Here's the drawing with two shaded views (mm, measured from the low corner). I have some questions. A direction names the side the tool comes from. Coordinates: 2 decimals unless noted, no trailing zeros. Write each loop counter-clockwise with the first axis right and the second up, starting at its lowest first coordinate (ties: lowest second). Pieces come first, ordered by that corner, then holes. Notation, with made-up numbers: (18.25, -17.75) -> (31.25, -17.75) arc R24 ccw to (31.25, 10.25) -> close; hole circle Ø4 at (76, 8). An arc over 180 degrees is marked (long way). Use one line per item in the form item = value.
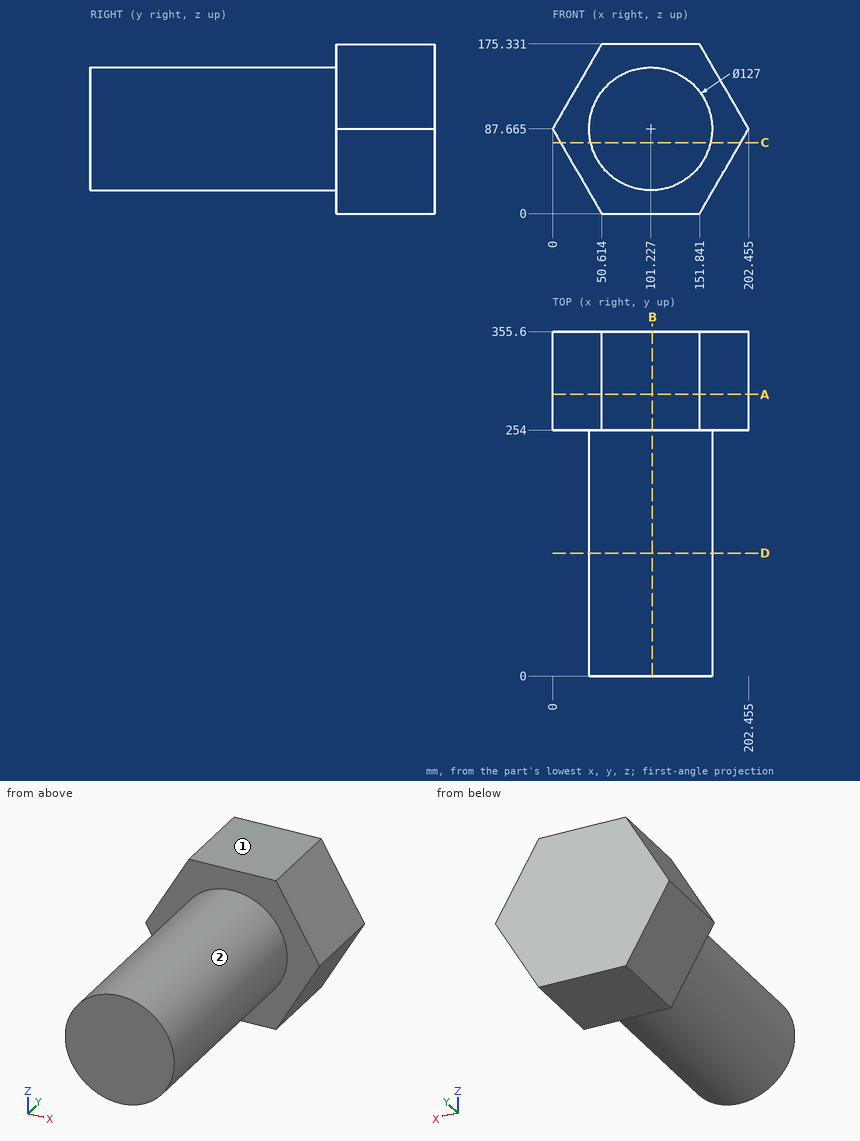
Q1. Suppose I cut it at B-B (x = 103). Write out the boundary of the cut face in (y, z).
Return value:
outline = (0, 24.19) -> (254, 24.19) -> (254, 0) -> (355.6, 0) -> (355.6, 175.33) -> (254, 175.33) -> (254, 151.14) -> (0, 151.14) -> close
Q2. If I drill on line 1 (Y direction, x = 31, z = 96); line 2 (Z direction, x = 127, y = 101); line 3 (X direction, y = 303, z = 164.5) (1 decimal), over which ranges is the centre line in solid material (lowest first)? Write a range as from..to.
Return value:
line_1 = 254..355.6
line_2 = 29.63..145.7
line_3 = 44.4..158.1
Q3. Suppose I cut it at C-C (z = 73.5). Write out the boundary of the cut face in (x, y).
Return value:
outline = (8.18, 254) -> (39.33, 254) -> (39.33, 0) -> (163.13, 0) -> (163.13, 254) -> (194.28, 254) -> (194.28, 355.6) -> (8.18, 355.6) -> close
Q4. Will these pins go through, and if not, where does the flat tip stop? pin 1 (6 mm diameter, centred on y = 84, z = 96, fed in from -X); pin 2 (6 mm diameter, centred on y = 289, z = 142, fed in from -X); pin 3 (6 mm diameter, centred on y = 316.5, z = 156, fed in from -X).
Return value:
pin_1 = 37.95
pin_2 = 29.64
pin_3 = 37.72
Q5. Suppose I cut it at D-D (y = 127). Write out the boundary of the cut face in (x, z) (1 decimal).
Return value:
outline = circle Ø127 at (101.2, 87.7)
Q6. For the marked faces 1 and 2, which set-ups out of +Z, -Z, +X, -X, +Y, -Y let a thin tool reach every point of the face, with its end or its side?
Return value:
face_1 = +Z, +X, -X, +Y, -Y
face_2 = -Y
Q7. Suppose I cut it at A-A (y = 291). Write out the boundary of the cut face in (x, z) (1 decimal), then the cut area to 3 significant figures.
Return value:
outline = (0, 87.7) -> (50.6, 0) -> (151.8, 0) -> (202.5, 87.7) -> (151.8, 175.3) -> (50.6, 175.3) -> close
area = 26,600 mm2
